Autodesk Inventor part; units mm, degrees
ref_plane "YZ Plane" through (0, 0, 0) normal (1, 0, 0) x (0, 1, 0)
ref_plane "XZ Plane" through (0, 0, 0) normal (0, 1, 0) x (-1, 0, 0)
ref_plane "XY Plane" through (0, 0, 0) normal (0, 0, 1) x (1, 0, 0)
sketch "스케치1" plane through (0, 0, 0) normal (0, 1, 0) x (-1, 0, 0)
  arc A0 (0, 5.25) -> (0, -5.25) centre (0, 0) ccw
  line L0 (0, 0) -> (0, 5.25) construction
  line L1 (0, 0) -> (5.25, 0) construction
  line L2 (0, 0) -> (0, -5.25) construction
  arc A1 (-2, 6.9687) -> (-2, -6.9687) centre (0, 0) ccw
  line L3 (0, 0) -> (0, -9) construction
  line L4 (0, 0) -> (0, 9) construction
  line L5 (0, 5.25) -> (0, 13.57)
  line L6 (0, 13.57) -> (-2, 13.57)
  line L7 (-2, 13.57) -> (-2, 6.9687)
  line L8 (0, -5.25) -> (0, -13.57)
  line L9 (0, -13.57) -> (-2, -13.57)
  line L10 (-2, -13.57) -> (-2, -6.9687)
  point P0 (-1, -13.57)
  point P1 (-1, 13.57)
  dimension "d46" = 5.25
  dimension "d47" = 90
  dimension "d48" = 180
  dimension "d49" = 7.25
  dimension "d50" = 180
  dimension "d51" = 13.57
  dimension "d52" = 13.57
  dimension "d53" = 2
  dimension "d54" = 2
extrude "돌출1" add sketch "스케치1" along normal blind 36.4
sketch "스케치2" plane through (2, 0, 13.57) normal (1, 0, 0) x (0, 0, -1)
  line L0 (0, 0) -> (6.6013, 0)
  line L1 (6.6013, 0) -> (6.6013, 36.4)
  line L2 (0, 36.4) -> (6.6013, 36.4)
  line L3 (0, 0) -> (0, 36.4)
  circle A0 centre (3.4, 26.75) radius 1.7
  circle A1 centre (3.4, 16.75) radius 1.7
  point P0 (13.57, 0)
  point P1 (3.3007, 36.4)
  dimension "d57" = 3.4
  dimension "d58" = 3.4
  dimension "d60" = 26.75
  dimension "d61" = 16.75
  dimension "d64" = 3.4
extrude "돌출2" cut sketch "스케치2" against normal through all contours A0 | A1
mirror "미러2" about plane through (0, 0, 0) normal (0, 0, 1) of "돌출2"
properties part number "pen고정부"
Geometry check sheet. Reference: the model listing, model coordinates, mm. A direction names the side the tool comes from. Round coordinates to 2 decimals unless told otherwise and drop trailing zeros. Write each loop counter-clockwise with the first axis right and the second up, starting at its lowest first coordinate (ties: lowest second). Pieces come first, ordered by that corner, then holes.
Item 1: Section check D-D (y = 3.5). Record the boundary of the cut face in (x, z), plus the area to 3 significant figures.
Determined:
outline: (0, -13.57) - (2, -13.57) - (2, -6.97) arc R7.25 ccw to (2, 6.97) - (2, 13.57) - (0, 13.57) - (0, 5.25) arc R5.25 cw to (0, -5.25) - close
area: 64.9 mm2
Item 2: Section check B-B (z = -10.17). Record the boundary of the cut face in (x, y).
Determined:
outline: (0, 0) - (2, 0) - (2, 15.05) - (0, 15.05) - close; (0, 18.45) - (2, 18.45) - (2, 25.05) - (0, 25.05) - close; (0, 28.45) - (2, 28.45) - (2, 36.4) - (0, 36.4) - close
Item 3: Go/stop test with flat-tipped pins: pin 1 Ø3.5 at (y, z) = (11.5, -9.5) entering from +X; pin 2 Ø2 at (y, z) = (16.75, -10.17) entering from -X; pin 3 Ø1 at (y, z) = (30, 2.5) entering from +X; pin 4 Ø6 at (y, z) = (8.5, -7.5) entering from +X. Record where each tip stops, or that it passes through.
Determined:
pin 1: stops at x = 2
pin 2: passes through
pin 3: stops at x = 6.97
pin 4: stops at x = 5.68
Item 4: Mould release check, pull along Z, two halves, no side actions. Record for faces 1 (the face through (0, 18, -8)), 2 (the face through (1, 17.4, -8.6)), 3 (the face through (7.25, 17.95, -0.13)): +Z half, -Z half, draft (parallel to the pull), parting line (faces both ways), or undercut.
Determined:
face 1: draft
face 2: undercut
face 3: parting line
Item 5: Material ranges on line 1 along Y through (x, z) = (1.3, 10.17); line 2 along Z through (x, y) = (1, 27.5); line 3 along X through (y, z) = (6, 12), recorded low to high.
Determined:
line 1: y = 0 to 15.05, 18.45 to 25.05, 28.45 to 36.4
line 2: z = -13.57 to -11.7, -8.64 to -5.15, 5.15 to 8.64, 11.7 to 13.57
line 3: x = 0 to 2
Item 6: Section check C-C (x = 3). Record the boundary of the cut face in (y, z).
Determined:
outline: (0, -6.6) - (36.4, -6.6) - (36.4, -4.31) - (0, -4.31) - close; (0, 4.31) - (36.4, 4.31) - (36.4, 6.6) - (0, 6.6) - close
Item 7: Access from +Z, -Z, +X, -X, +Y, -Y to the whole of each face (thin tool, end or side, straight path). Record for faces 4 (the face through (2, 18, -12)), 5 (the face through (1, 18, 13.57)), 6 (the face through (2, 18, 12)).
Determined:
face 4: -Z, +X, +Y, -Y
face 5: +Z, +X, -X, +Y, -Y
face 6: +Z, +X, +Y, -Y
Item 8: Section check A-A (y = 16.75). Record the boundary of the cut face in (x, z).
Determined:
outline: (0, -13.57) - (2, -13.57) - (2, -11.87) - (0, -11.87) - close; (0, -8.47) - (2, -8.47) - (2, -6.97) arc R7.25 ccw to (2, 6.97) - (2, 8.47) - (0, 8.47) - (0, 5.25) arc R5.25 cw to (0, -5.25) - close; (0, 11.87) - (2, 11.87) - (2, 13.57) - (0, 13.57) - close
